Design review of the part shown in the three views and the two pictorial views. Dimensions are in mm from the part's minimum x, y and z. A direction names the side the tool comes from. Round coordinates to 2 decimals unless told otherwise and drop trailing zeros. Order: outer loops, then holes, each group sorted by start corner. A loop starts at its lowest first (then second) coordinate and runs counter-clockwise, first axis right, second up. Notation, with made-up numbers: M 80,19 L 92,19 A25 cw 92,57 Z; hole C -19,84 d2. An arc over 180 degrees is marked long. Use a Markdown table: item, result. Add a question column.
(1) To check wall thickness, follow probe 1 along Y at (x, z) = (2.5, 29); probe 2 along Z at (x, y) = (78, 9.25); probe 3 along X at (y, z) = (3.25, 21.5). State the ranges of each line that lie inside material, in increasing order. Write a range as from..to.
(2) Machinability: for the marked faces 1, 2, 3 and 4, which of the approach directions +Z, -Z, +X, -X, +Y, -Y give a long, thin tool a straight path to every point of the face, cutting with its end or side? Answer none if there is none.
(3) Take a section at B-B (y = 15.5). Write out the cut boundary in (x, z).
(4) Take a section at A-A (x = 97.5). Write out the cut boundary in (y, z).
(5) Take a section at D-D (z = 6). Write out the cut boundary in (x, y).
(6) Take a section at C-C (y = 7.25). Write out the cut boundary in (x, z), then the cut area to 3 significant figures.
(7) For pin 1 (12 mm diameter, centred on x = 20, y = 6.5, fed in from -Z); pin 2 (1 mm diameter, centred on y = 8.5, z = 23.5, fed in from +X); pin 3 (1 mm diameter, centred on x = 49.5, y = 7.5, fed in from -Z); pin 4 (6 mm diameter, centred on x = 28, y = 9.5, fed in from -Z), all flat-tipped, find the tip position at first contact; note any pin that passes through.
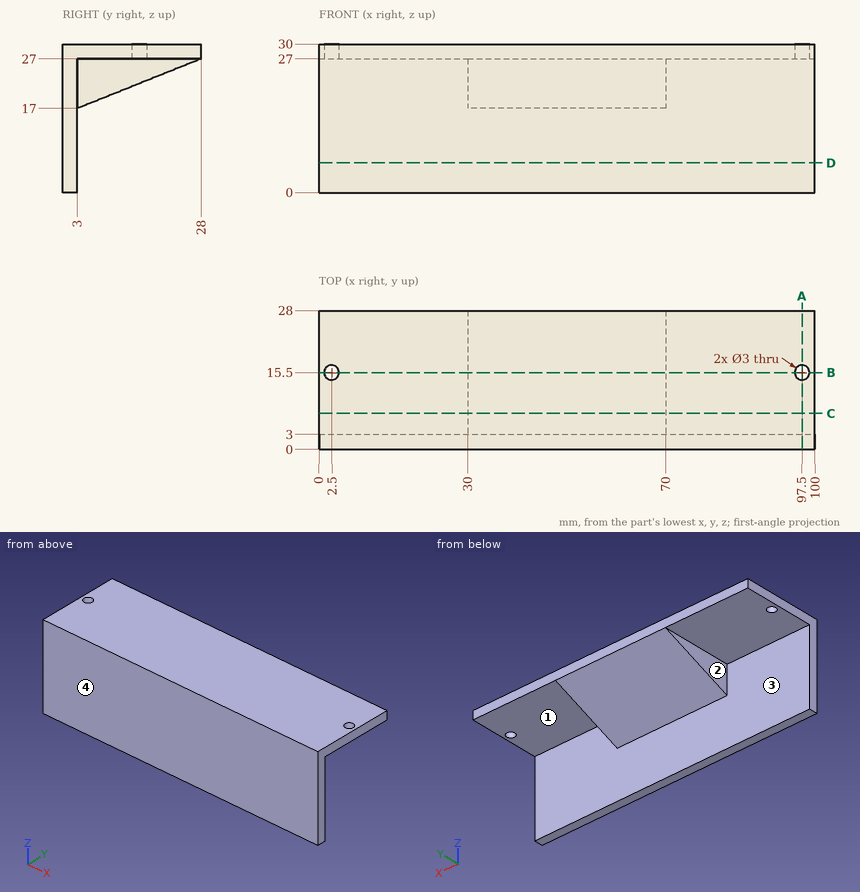
Verdict:
| question | item | result |
|---|---|---|
| 1 | probe 1 | y = 0..14, 17..28 |
| 1 | probe 2 | z = 27..30 |
| 1 | probe 3 | x = 30..70 |
| 2 | face 1 | -Z, +X, +Y |
| 2 | face 2 | -Z, -X, +Y |
| 2 | face 3 | -Z, +Y |
| 2 | face 4 | +Z, -Z, +X, -X, -Y |
| 3 | outline | M 0,27 L 1,27 L 1,30 L 0,30 Z; M 4,27 L 30,27 L 30,22 L 70,22 L 70,27 L 96,27 L 96,30 L 4,30 Z; M 99,27 L 100,27 L 100,30 L 99,30 Z |
| 4 | outline | M 0,0 L 3,0 L 3,27 L 14,27 L 14,30 L 0,30 Z; M 17,27 L 28,27 L 28,30 L 17,30 Z |
| 5 | outline | M 0,0 L 100,0 L 100,3 L 0,3 Z |
| 6 | outline | M 0,27 L 30,27 L 30,18.7 L 70,18.7 L 70,27 L 100,27 L 100,30 L 0,30 Z |
| 6 | area | 632 mm^2 |
| 7 | pin 1 | stops at z = 0 |
| 7 | pin 2 | stops at x = 70 |
| 7 | pin 3 | stops at z = 18.6 |
| 7 | pin 4 | stops at z = 18.71 |
